Could you check a few things on this model? Use its own coordinates, in mm. Give positions to 0.01 mm unless a question says otherwise; leave off trailing zeros. Write item = value, one per line. Start each with the question number.
Autodesk Inventor part; units mm, degrees
ref_plane "YZ Plane" through (0, 0, 0) normal (1, 0, 0) x (0, 1, 0)
ref_plane "XZ Plane" through (0, 0, 0) normal (0, 1, 0) x (-1, 0, 0)
ref_plane "XY Plane" through (0, 0, 0) normal (0, 0, 1) x (1, 0, 0)
sketch "Sketch1" plane through (0, 0, 0) normal (0, 0, 1) x (1, 0, 0)
  line L0 (-152.4, 304.8) -> (152.4, 304.8)
  line L1 (152.4, 304.8) -> (152.4, 0)
  line L2 (152.4, 0) -> (-152.4, 0)
  line L3 (-152.4, 0) -> (-152.4, 304.8)
  point P0 (0, 0)
  point P1 (0, 0)
extrude "Extrusion1" add sketch "Sketch1" along normal mid plane 304.8
sketch "Sketch2" plane through (0, 0, 152.4) normal (0, 0, 1) x (1, 0, 0)
  line L0 (-152.4, 304.8) -> (152.4, 304.8)
  line L1 (-3.175, 304.8) -> (3.175, 304.8)
  line L2 (3.175, 304.8) -> (3.175, 301.625)
  line L3 (3.175, 301.625) -> (-3.175, 301.625)
  line L4 (-3.175, 301.625) -> (-3.175, 304.8)
  point P0 (0, 0)
  point P1 (0, 304.8)
  dimension "d4" = 3.175
  dimension "d5" = 6.35
extrude "Extrusion2" cut sketch "Sketch2" against normal through all
sketch "Sketch3" plane through (0, 0, 152.4) normal (0, 0, 1) x (1, 0, 0)
  line L0 (-152.4, 0) -> (-152.4, 304.8)
  line L1 (152.4, 0) -> (-152.4, 0)
  line L2 (-127, 25.4) -> (-50.8, 25.4)
  line L3 (-50.8, 25.4) -> (-50.8, 101.6)
  line L4 (-50.8, 101.6) -> (-127, 101.6)
  line L5 (-127, 101.6) -> (-127, 25.4)
  line L6 (-123.825, 98.425) -> (-53.975, 98.425)
  line L7 (-53.975, 98.425) -> (-53.975, 28.575)
  line L8 (-53.975, 28.575) -> (-123.825, 28.575)
  line L9 (-123.825, 28.575) -> (-123.825, 98.425)
  line L10 (-38.1, 25.4) -> (38.1, 25.4)
  line L11 (38.1, 25.4) -> (38.1, 101.6)
  line L12 (38.1, 101.6) -> (-38.1, 101.6)
  line L13 (-38.1, 101.6) -> (-38.1, 25.4)
  line L14 (-34.925, 98.425) -> (34.925, 98.425)
  line L15 (34.925, 98.425) -> (34.925, 28.575)
  line L16 (34.925, 28.575) -> (-34.925, 28.575)
  line L17 (-34.925, 28.575) -> (-34.925, 98.425)
  line L18 (-127, 114.3) -> (-50.8, 114.3)
  line L19 (-50.8, 114.3) -> (-50.8, 190.5)
  line L20 (-50.8, 190.5) -> (-127, 190.5)
  line L21 (-127, 190.5) -> (-127, 114.3)
  line L22 (-123.825, 187.325) -> (-53.975, 187.325)
  line L23 (-53.975, 187.325) -> (-53.975, 117.475)
  line L24 (-53.975, 117.475) -> (-123.825, 117.475)
  line L25 (-123.825, 117.475) -> (-123.825, 187.325)
  line L26 (-38.1, 114.3) -> (38.1, 114.3)
  line L27 (38.1, 114.3) -> (38.1, 190.5)
  line L28 (38.1, 190.5) -> (-38.1, 190.5)
  line L29 (-38.1, 190.5) -> (-38.1, 114.3)
  line L30 (-34.925, 187.325) -> (34.925, 187.325)
  line L31 (34.925, 187.325) -> (34.925, 117.475)
  line L32 (34.925, 117.475) -> (-34.925, 117.475)
  line L33 (-34.925, 117.475) -> (-34.925, 187.325)
  point P0 (0, 0)
  dimension "d8" = 76.2
  dimension "d9" = 25.4
  dimension "d10" = 25.4
  dimension "d11" = 3.175
  dimension "d14" = 88.9
  dimension "d17" = 88.9
split_face "Split1"
split_face "Split2"
split_face "Split3"
split_face "Split4"
split_face "Split5"
split_face "Split6"
split_face "Split7"
split_face "Split8"
sketch "Sketch4" plane through (-123.825, 98.425, 152.4) normal (0, 0, 1) x (1, 0, 0)
  line L0 (0, 0) -> (69.85, 0)
  line L1 (0, -69.85) -> (0, 0)
  line L2 (69.85, -69.85) -> (0, -69.85)
  line L3 (19.0891, -57.15) -> (50.7609, -57.15)
  line L4 (50.7609, -57.15) -> (50.7609, -50.8)
  line L5 (19.0891, -50.8) -> (19.0891, -57.15)
  line L6 (38.1, -50.8) -> (38.1, -34.697)
  line L7 (31.75, -34.697) -> (31.75, -50.8)
  line L8 (19.6575, -12.7) -> (16.6521, -18.8843)
  line L9 (16.6521, -18.8843) -> (20.9342, -18.8843)
  line L10 (20.9342, -18.8843) -> (17.3368, -26.287)
  line L11 (22.15, -12.7) -> (20.3175, -16.4708)
  line L12 (20.3175, -16.4708) -> (24.6183, -16.4708)
  line L13 (24.6183, -16.4708) -> (18.9446, -28.1459)
  line L14 (12.7, -12.7) -> (19.6575, -12.7)
  line L15 (22.15, -12.7) -> (57.15, -12.7)
  arc A0 (12.7, -12.7) -> (17.3368, -26.287) centre (34.925, -12.7) ccw
  arc A1 (18.9446, -28.1459) -> (31.75, -34.697) centre (34.925, -12.7) ccw
  arc A2 (38.1, -34.697) -> (57.15, -12.7) centre (34.925, -12.7) ccw
  line L16 (50.7609, -50.8) -> (38.1, -50.8)
  line L17 (31.75, -50.8) -> (19.0891, -50.8)
  point P0 (123.825, -98.425)
  point P1 (34.925, -50.8)
  point P2 (34.925, -29.1715)
  point P3 (34.925, 0)
  dimension "d20" = 12.7
  dimension "d21" = 6.35
  dimension "d22" = 6.35
  dimension "d24" = 12.7
split_face "Split9"
split_face "Split10"
sketch "Sketch5" plane through (-34.925, 98.425, 152.4) normal (0, 0, 1) x (1, 0, 0)
  line L0 (69.85, 0) -> (69.85, -69.85)
  line L1 (0, 0) -> (69.85, 0)
  line L2 (0, -69.85) -> (0, 0)
  line L3 (69.85, -69.85) -> (0, -69.85)
  line L4 (57.15, -12.7) -> (57.15, -57.15) construction
  line L5 (57.15, -57.15) -> (12.7, -57.15) construction
  line L6 (12.7, -57.15) -> (12.7, -12.7) construction
  line L7 (12.7, -12.7) -> (57.15, -12.7) construction
  line L8 (36.0188, -31.0952) -> (36.0188, -51.4628)
  line L9 (33.8312, -51.4628) -> (33.8312, -31.0952)
  arc A0 (24.6443, -51.4628) -> (36.0188, -51.4628) centre (30.3316, -51.4628) ccw
  arc A1 (26.8319, -51.4628) -> (33.8312, -51.4628) centre (30.3316, -51.4628) ccw
  line L10 (24.6443, -51.4628) -> (26.8319, -51.4628)
  line L11 (36.0188, -13.8321) -> (36.0188, -12.7)
  line L12 (36.0188, -12.7) -> (33.8312, -12.7)
  line L13 (33.8312, -12.7) -> (33.8312, -13.8301)
  arc A2 (23.1675, -30.5813) -> (12.7, -30.0146) centre (17.5638, -37.131) ccw
  arc A3 (33.8312, -30.1527) -> (23.1675, -30.5813) centre (28.7712, -37.131) ccw
  arc A4 (46.5876, -30.5012) -> (36.0188, -30.1527) centre (41.0788, -37.131) ccw
  arc A5 (57.15, -30.1481) -> (46.5876, -30.5012) centre (52.0963, -37.131) ccw
  line L14 (36.0188, -31.0952) -> (36.0188, -30.1527)
  line L15 (33.8312, -31.0952) -> (33.8312, -30.1527)
  arc A6 (57.15, -30.1481) -> (36.0188, -13.8321) centre (34.9039, -37.1178) ccw
  arc A7 (33.8312, -13.8301) -> (12.7, -30.0146) centre (34.9039, -37.1178) ccw
  point P0 (34.925, -98.425)
  point P1 (34.925, -31.0952)
  point P2 (34.925, -31.0952)
  point P3 (34.925, -12.7)
  dimension "d25" = 12.7
split_face "Split11"
sketch "Sketch6" plane through (-34.925, 187.325, 152.4) normal (0, 0, 1) x (1, 0, 0)
  line L0 (69.85, 0) -> (69.85, -69.85)
  line L1 (0, 0) -> (69.85, 0)
  line L2 (0, -69.85) -> (0, 0)
  line L3 (69.85, -69.85) -> (0, -69.85)
  line L4 (57.15, -12.7) -> (57.15, -57.15) construction
  line L5 (57.15, -57.15) -> (12.7, -57.15)
  line L6 (12.7, -57.15) -> (12.7, -12.7) construction
  line L7 (12.7, -12.7) -> (57.15, -12.7) construction
  line L8 (12.7, -50.8) -> (57.15, -50.8)
  line L9 (22.6976, -12.7) -> (17.5193, -23.9944)
  line L10 (27.8758, -23.9944) -> (22.6976, -12.7)
  line L11 (25.8726, -23.9944) -> (25.8726, -48.0363)
  line L12 (25.8726, -48.0363) -> (19.5226, -48.0363)
  line L13 (19.5226, -48.0363) -> (19.5226, -23.9944)
  line L14 (34.925, -12.7) -> (34.925, -7.7199) construction
  line L15 (47.1524, -12.7) -> (52.3307, -23.9944)
  line L16 (41.9742, -23.9944) -> (47.1524, -12.7)
  line L17 (43.9774, -23.9944) -> (43.9774, -48.0363)
  line L18 (43.9774, -48.0363) -> (50.3274, -48.0363)
  line L19 (50.3274, -48.0363) -> (50.3274, -23.9944)
  line L20 (12.7, -50.8) -> (12.7, -57.15)
  line L21 (57.15, -50.8) -> (57.15, -57.15)
  line L22 (17.5193, -23.9944) -> (19.5226, -23.9944)
  line L23 (25.8726, -23.9944) -> (27.8758, -23.9944)
  line L24 (52.3307, -23.9944) -> (50.3274, -23.9944)
  line L25 (43.9774, -23.9944) -> (41.9742, -23.9944)
  point P0 (34.925, -187.325)
  point P1 (22.6976, -23.9944)
  point P2 (47.1524, -23.9944)
  dimension "d26" = 12.7
  dimension "d27" = 6.35
  dimension "d28" = 6.35
split_face "Split12"
split_face "Split13"
split_face "Split14"
sketch "Sketch7" plane through (-123.825, 187.325, 152.4) normal (0, 0, 1) x (1, 0, 0)
  line L0 (0, -69.85) -> (69.85, -69.85)
  line L1 (12.7, -12.7) -> (57.15, -12.7) construction
  line L2 (57.15, -57.15) -> (12.7, -57.15) construction
  line L3 (22.6688, -57.15) -> (22.6688, -52.8524)
  arc A0 (22.6688, -52.8524) -> (20.3647, -47.1054) centre (14.3497, -52.8524) ccw
  line L4 (20.3647, -47.1054) -> (15.1508, -41.6484)
  arc A1 (12.7, -34.925) -> (15.1508, -41.6484) centre (21.5956, -35.4908) ccw
  line L5 (15.875, -19.6032) -> (15.875, -31.6397)
  line L6 (17.6337, -36.0264) -> (26.3364, -45.1349)
  arc A2 (26.3364, -45.1349) -> (28.0331, -43.5138) centre (27.1847, -44.3243) ccw
  line L7 (28.0331, -43.5138) -> (21.521, -36.698)
  arc A3 (23.8166, -34.5047) -> (21.521, -36.698) centre (22.6688, -35.6013) ccw
  line L8 (23.8166, -34.5047) -> (30.3287, -41.3205)
  arc A4 (31.533, -44.3243) -> (30.3287, -41.3205) centre (27.1847, -44.3243) ccw
  line L9 (31.533, -44.3243) -> (31.533, -57.15)
  line L10 (34.925, -12.7) -> (34.925, -57.15) construction
  arc A5 (15.875, -19.6032) -> (12.7, -19.6032) centre (14.2875, -19.6032) ccw
  arc A6 (15.875, -31.6397) -> (17.6337, -36.0264) centre (22.225, -31.6397) ccw
  line L11 (12.7, -34.925) -> (12.7, -19.6032)
  line L12 (47.1812, -57.15) -> (47.1812, -52.8524)
  arc A7 (49.4853, -47.1054) -> (47.1812, -52.8524) centre (55.5003, -52.8524) ccw
  line L13 (49.4853, -47.1054) -> (54.6992, -41.6484)
  arc A8 (54.6992, -41.6484) -> (57.15, -34.925) centre (48.2544, -35.4908) ccw
  line L14 (53.975, -19.6032) -> (53.975, -31.6397)
  line L15 (52.2163, -36.0264) -> (43.5136, -45.1349)
  arc A9 (41.8169, -43.5138) -> (43.5136, -45.1349) centre (42.6653, -44.3243) ccw
  line L16 (41.8169, -43.5138) -> (48.329, -36.698)
  arc A10 (48.329, -36.698) -> (46.0334, -34.5047) centre (47.1812, -35.6013) ccw
  line L17 (46.0334, -34.5047) -> (39.5213, -41.3205)
  arc A11 (39.5213, -41.3205) -> (38.317, -44.3243) centre (42.6653, -44.3243) ccw
  line L18 (38.317, -44.3243) -> (38.317, -57.15)
  arc A12 (57.15, -19.6032) -> (53.975, -19.6032) centre (55.5625, -19.6032) ccw
  arc A13 (52.2163, -36.0264) -> (53.975, -31.6397) centre (47.625, -31.6397) ccw
  line L19 (38.317, -57.15) -> (47.1812, -57.15)
  line L20 (57.15, -19.6032) -> (57.15, -34.925)
  line L21 (34.925, -12.7) -> (26.384, -18.361)
  line L22 (26.384, -18.361) -> (34.925, -24.0221)
  line L23 (34.925, -24.0221) -> (43.466, -18.361)
  line L24 (43.466, -18.361) -> (34.925, -12.7)
  line L25 (26.5258, -20.3104) -> (33.8787, -25.1839)
  line L26 (33.8787, -25.1839) -> (33.8787, -33.5217)
  line L27 (33.8787, -33.5217) -> (26.5258, -28.6482)
  line L28 (26.5258, -28.6482) -> (26.5258, -20.3104)
  line L29 (43.3242, -20.3104) -> (35.9713, -25.1839)
  line L30 (35.9713, -25.1839) -> (35.9713, -33.5217)
  line L31 (35.9713, -33.5217) -> (43.3242, -28.6482)
  line L32 (43.3242, -28.6482) -> (43.3242, -20.3104)
  line L33 (22.6688, -57.15) -> (31.533, -57.15)
  line L34 (57.15, -12.7) -> (57.15, -34.925) construction
  line L35 (57.15, -36.0566) -> (57.15, -57.15) construction
  line L36 (12.7, -57.15) -> (12.7, -36.0566) construction
  line L37 (12.7, -34.925) -> (12.7, -12.7) construction
  point P0 (123.825, -187.325)
  dimension "d30" = 12.7
  dimension "d32" = 3.175
  dimension "d33" = 6.35
split_face "Split15"
split_face "Split16"
split_face "Split17"
split_face "Split18"
split_face "Split19"
sketch "Sketch8" plane through (-152.4, 304.8, -152.4) normal (0, 1, 0) x (1, 0, 0)
  line L0 (149.225, -304.8) -> (149.225, 0)
  line L1 (149.225, 0) -> (0, 0)
  line L2 (0, 0) -> (0, -304.8)
  line L3 (0, -304.8) -> (149.225, -304.8)
  line L4 (0, 0) -> (304.8, -304.8)
  point P0 (152.4, -152.4)
sketch "Sketch9" plane through (0, 0, -152.4) normal (0, 0, -1) x (-1, 0, 0)
  line L0 (-3.175, 301.625) -> (-3.175, 304.8)
  line L1 (-152.4, 304.8) -> (-3.175, 304.8)
  line L2 (-152.4, 0) -> (-152.4, 304.8)
  line L3 (152.4, 0) -> (-152.4, 0)
  line L4 (152.4, 304.8) -> (152.4, 0)
  line L5 (3.175, 304.8) -> (152.4, 304.8)
  line L6 (3.175, 304.8) -> (3.175, 301.625)
  line L7 (3.175, 301.625) -> (-3.175, 301.625)
  line L8 (152.4, 304.8) -> (-152.4, 0)
  point P0 (0, 0)
  point P1 (0, 152.4)
sketch "Sketch10" plane through (-152.4, 0, 152.4) normal (0, 0, 1) x (1, 0, 0)
  line L0 (101.6, 25.4) -> (101.6, 101.6)
  line L1 (25.4, 25.4) -> (101.6, 25.4)
  line L2 (25.4, 101.6) -> (25.4, 25.4)
  line L3 (101.6, 101.6) -> (25.4, 101.6)
  line L4 (155.575, 304.8) -> (155.575, 301.625)
  line L5 (155.575, 301.625) -> (149.225, 301.625)
  line L6 (149.225, 301.625) -> (149.225, 304.8)
  line L7 (0, 304.8) -> (149.225, 304.8)
  line L8 (0, 0) -> (0, 304.8)
  line L9 (304.8, 0) -> (0, 0)
  line L10 (304.8, 304.8) -> (304.8, 0)
  line L11 (155.575, 304.8) -> (304.8, 304.8)
  line L12 (101.6, 190.5) -> (101.6, 114.3)
  line L13 (101.6, 114.3) -> (25.4, 114.3)
  line L14 (25.4, 114.3) -> (25.4, 190.5)
  line L15 (25.4, 190.5) -> (101.6, 190.5)
  line L16 (190.5, 114.3) -> (190.5, 190.5)
  line L17 (114.3, 114.3) -> (190.5, 114.3)
  line L18 (114.3, 190.5) -> (114.3, 114.3)
  line L19 (190.5, 190.5) -> (114.3, 190.5)
  line L20 (190.5, 25.4) -> (190.5, 101.6)
  line L21 (114.3, 25.4) -> (190.5, 25.4)
  line L22 (114.3, 101.6) -> (114.3, 25.4)
  line L23 (190.5, 101.6) -> (114.3, 101.6)
  line L24 (0, 304.8) -> (304.8, 0)
  point P0 (152.4, 0)
  point P1 (152.4, 152.4)
equation "\"d28\" = d27"
equation "\"d32\" = d31"
properties part number "Box - Package"
(1) If I drill on line 1 along Y through (x, z) = (-2.5, 7.5) (3 decimals), over which ranges is the centre line in solid material (lowest first)? Write a range as from..to.
(2) We'd pull the mould along X, two halves only. Please class faces 1 (the flat face through (152.4, 155, -2)), 2 (the flat face through (-152.4, 150, -2)), 3 (the flat face through (-2, 155, 152.4)): released by +X, released by -X, zero draft, split by the parting line, or undercut.
(3) I'm going to push a flat-ended pin straight in: pin 1 (1 mm diameter, centred on x = -10, z = -65.5, fed in from -Y). Where does the tip first touch, or does it pass through?
Answers below:
q1.line_1 = 0..301.625
q2.face_1 = released by +X
q2.face_2 = released by -X
q2.face_3 = zero draft
q3.pin_1 = 0
